Model file for the job. Use its own axes, mm. Give positions to 0.01 mm unless a question says otherwise; leave off trailing zeros. Order: outer loops, then holes, each group sorted by start corner. A loop starts at its lowest first (then second) coordinate and runs counter-clockwise, first axis right, second up. Notation, with made-up numbers: (72, 56.25) - (112, 56.25) arc R9 cw to (112, 63.25) - close; hole circle Ø6 at (-13.5, 44.5). An arc over 180 degrees is marked (long way). Use CSV: the item, a comma, the result in double quotes. Start each with the question number.
(1) Band-saw the part on D-D, the plane x = -13.5. Give the cut face in (y, z).
(2) Probe L1, parallel to X at y = 18, z = 2.15; L2, parallel to Y at x = 0, z = 2.2; L3, parallel to Y at x = -14, z = 2.4. List the from-to ranges inside material, lowest first.
(3) Band-saw the part on A-A, the plane x = 0. Give the cut face in (y, z), then the cut area to 3 significant figures.
(4) Drop flat-ended pins along their axis: pin 1 Ø2.5 at (x, y) = (0, 0) entering from +Z; pin 2 Ø1 at (y, z) = (-2, 2) entering from +X. Give the stop position or say it passes through.
(5) Band-saw the part on C-C, the plane z = 1.75. Give the cut face in (x, y), then the cut area to 3 significant figures.
(6) Band-saw the part on B-B, the plane y = 0. Give the cut face in (x, z), then the cut area to 3 significant figures.
(7) Pull direction Y, two halves, no side cores. Call faces 1 (the cylindrical face through (-30.484, -1.273, 1.479)), 2 (the cylindrical face through (-5.455, 18.219, 1.479)), 3 (the flat face through (6.193, 12.023, 1.521)): +Y half, -Y half, draft (parallel to the pull), parting line (faces both ways), or undercut.
from build123d import *

# Parameters (mm, degrees)
SCHIZZO1_W                   = 46
SCHIZZO1_H                   = 38
SCHIZZO1_R                   = 1.5
ESTRUSIONE_ESTRUSIONE3_DEPTH = 3
TAGLIO_ESTRUSIONE1_DEPTH     = 3
RACCORDO1_R                  = 15
RACCORDO2_R                  = 15
RACCORDO3_R                  = 20
RACCORDO4_R                  = 20


with BuildPart() as part:
    # Schizzo1 → Estrusione-Estrusione3 (new body)
    with BuildSketch(Plane.XY):
        with Locations((-10.000402867, 5)):
            Rectangle(SCHIZZO1_W, SCHIZZO1_H)
        with Locations((-6.840402867, 18.793852416)):
            Circle(SCHIZZO1_R, mode=Mode.SUBTRACT)
        Circle(SCHIZZO1_R, mode=Mode.SUBTRACT)
        with Locations((-20.000805733, 0)):
            Circle(SCHIZZO1_R, mode=Mode.SUBTRACT)
        with Locations((-13.160402867, 18.793852416)):
            Circle(SCHIZZO1_R, mode=Mode.SUBTRACT)
    extrude(amount=ESTRUSIONE_ESTRUSIONE3_DEPTH)

    # Schizzo4 → Taglio-Estrusione1 (cut)
    with BuildSketch(Plane.XY.offset(3)):
        Polygon((-33.000402867, -1.13961018), (-20.000402867, 24), (-33.000402867, 24), align=None)
        Polygon((12.999597133, 24), (-0.000402867, 24), (12.999597133, -1.13961018), align=None)
        Polygon((-26.350137947, -14), (-33.000402867, -1.13961018), (-33.000402867, -14), align=None)
        Polygon((12.999597133, -14), (12.999597133, -1.13961018), (6.349332214, -14), align=None)
    extrude(amount=-TAGLIO_ESTRUSIONE1_DEPTH, mode=Mode.SUBTRACT)

    # Raccordo1
    raccordo1_edges = [part.edges().sort_by_distance(p)[0] for p in [
        (-0.000402867, 24, 1.5),
    ]]
    fillet(raccordo1_edges, radius=RACCORDO1_R)

    # Raccordo2
    raccordo2_edges = [part.edges().sort_by_distance(p)[0] for p in [
        (-20.000402867, 24, 1.5),
    ]]
    fillet(raccordo2_edges, radius=RACCORDO2_R)

    # Raccordo3
    raccordo3_edges = [part.edges().sort_by_distance(p)[0] for p in [
        (12.999597133, -1.13961018, 1.5),
    ]]
    fillet(raccordo3_edges, radius=RACCORDO3_R)

    # Raccordo4
    raccordo4_edges = [part.edges().sort_by_distance(p)[0] for p in [
        (-33.000402867, -1.13961018, 1.5),
    ]]
    fillet(raccordo4_edges, radius=RACCORDO4_R)


solid = part.part
Answer block:
1,outline,"(-14, 0) - (17.33, 0) - (17.33, 3) - (-14, 3) - close; (20.25, 0) - (23.77, 0) - (23.77, 3) - (20.25, 3) - close"
2,L1,"x = -22.87 to -14.43, -11.89 to -8.11, -5.57 to 2.87"
2,L2,"y = -14 to -1.5, 1.5 to 20.9"
2,L3,"y = -14 to 17.55, 20.04 to 23.67"
3,outline,"(-14, 0) - (-1.5, 0) - (-1.5, 3) - (-14, 3) - close; (1.5, 0) - (20.9, 0) - (20.9, 3) - (1.5, 3) - close"
3,area,"95.7 mm2"
4,pin 1,"passes through"
4,pin 2,"stops at x = 10.48"
5,outline,"(-28.25, -10.33) - (-26.35, -14) - (6.35, -14) - (8.25, -10.33) arc R20 ccw to (8.25, 8.05) - (4.19, 15.89) arc R15 ccw to (-9.13, 24) - (-10.87, 24) arc R15 ccw to (-24.19, 15.89) - (-28.25, 8.05) arc R20 ccw to start; hole circle Ø3 at (-20, 0); hole circle Ø3 at (-13.16, 18.79); hole circle Ø3 at (-6.84, 18.79); hole circle Ø3 at (0, 0)"
5,area,"1,250 mm2"
6,outline,"(-30.45, 0) - (-21.5, 0) - (-21.5, 3) - (-30.45, 3) - close; (-18.5, 0) - (-1.5, 0) - (-1.5, 3) - (-18.5, 3) - close; (1.5, 0) - (10.45, 0) - (10.45, 3) - (1.5, 3) - close"
6,area,"105 mm2"
7,face 1,"parting line"
7,face 2,"undercut"
7,face 3,"+Y half"
